Read the model definition and answer for the solid it produces. Units are mm, in the model's axes. A direction names the side the tool comes from. Coordinates: 2 decimals unless noted, no trailing zeros. Order: outer loops, then holes, each group sorted by start corner. A loop starts at its lowest first (then second) coordinate and runs counter-clockwise, first axis right, second up. Notation, with made-up numbers: (46, 50) -> (98, 50) arc R29 cw to (98, 74) -> close; hole circle Ø10 at (-35.5, -19.5). An arc over 180 degrees is marked (long way). Answer in a Markdown table with one row per item.
from build123d import *

# Parameters (mm, degrees)
FACE_SKETCH_W                       = 145.5
FACE_SKETCH_H                       = 95.5
FACE_SKETCH_R                       = 0.5
FACE_SKETCH_R_2                     = 2.5
FACE_SKETCH_R_3                     = 4
FACE_SKETCH_W_2                     = 80.6
FACE_SKETCH_H_2                     = 53.2
FACE_EXTRUDE_DEPTH                  = 2.25
SKETCH1_R                           = 11.375
STOP_BUTTON_MOUNTING_HOLE_CUT_DEPTH = 107.125809773
WALLS_SKETCH_W                      = 145.5
WALLS_SKETCH_H                      = 95.5
WALLS_SKETCH_W_2                    = 141
WALLS_SKETCH_H_2                    = 91
WALLS_EXTRUDE_DEPTH                 = 21.25
SD_CARD_ACCESS_SKETCH_W             = 9.5
SD_CARD_ACCESS_SKETCH_H             = 31
SD_CARD_CUT_DEPTH                   = 2.5
EDGE_RADIUS_R                       = 2
TOP_CONNECTORS_CUT_DEPTH            = 109.208999164
TOP_CONNECTORS_CUT_DEPTH_BACK       = 109.208999164
TOP_CONNECTORS_SKETCH_R             = 1.6


with BuildPart() as part:
    # Face Sketch → Face Extrude (new body)
    with BuildSketch(Plane.XY):
        with Locations((22, 0)):
            Rectangle(FACE_SKETCH_W, FACE_SKETCH_H)
        with Locations((18.7, -35.5)):
            Circle(FACE_SKETCH_R, mode=Mode.SUBTRACT)
        with Locations((3.5, -35.5)):
            Circle(FACE_SKETCH_R_2, mode=Mode.SUBTRACT)
        with Locations((36.5, -35.5)):
            Circle(FACE_SKETCH_R_3, mode=Mode.SUBTRACT)
        with Locations((18.7, -32)):
            Circle(FACE_SKETCH_R, mode=Mode.SUBTRACT)
        with Locations((21.731088913, -33.75)):
            Circle(FACE_SKETCH_R, mode=Mode.SUBTRACT)
        with Locations((21.731088913, -37.25)):
            Circle(FACE_SKETCH_R, mode=Mode.SUBTRACT)
        with Locations((18.7, -39)):
            Circle(FACE_SKETCH_R, mode=Mode.SUBTRACT)
        with Locations((15.668911087, -37.25)):
            Circle(FACE_SKETCH_R, mode=Mode.SUBTRACT)
        with Locations((15.668911087, -33.75)):
            Circle(FACE_SKETCH_R, mode=Mode.SUBTRACT)
        with Locations((0, 8.6)):
            Rectangle(FACE_SKETCH_W_2, FACE_SKETCH_H_2, mode=Mode.SUBTRACT)
    extrude(amount=FACE_EXTRUDE_DEPTH)

    # Sketch1 → Stop Button Mounting Hole Cut (cut, through all)
    with BuildSketch(Plane.XY):
        with Locations((72.75, 0)):
            Circle(SKETCH1_R)
    extrude(amount=STOP_BUTTON_MOUNTING_HOLE_CUT_DEPTH, mode=Mode.SUBTRACT)

    # Walls Sketch → Walls Extrude (add)
    with BuildSketch(Plane(origin=(0, 0, 0), x_dir=(-1, 0, 0), z_dir=(0, 0, -1))):
        with Locations((-22, 0)):
            Rectangle(WALLS_SKETCH_W, WALLS_SKETCH_H)
        with Locations((-22, 0)):
            Rectangle(WALLS_SKETCH_W_2, WALLS_SKETCH_H_2, mode=Mode.SUBTRACT)
    extrude(amount=WALLS_EXTRUDE_DEPTH)

    # SD Card Access Sketch → SD Card Cut (cut)
    with BuildSketch(Plane.ZY.offset(50.75)):
        with Locations((-16.5, 7.5)):
            Rectangle(SD_CARD_ACCESS_SKETCH_W, SD_CARD_ACCESS_SKETCH_H)
    extrude(amount=-SD_CARD_CUT_DEPTH, mode=Mode.SUBTRACT)

    # Edge Radius
    edge_radius_edges = [part.edges().sort_by_distance(p)[0] for p in [
        (94.75, 0, 2.25),
        (22, 47.75, 2.25),
        (-50.75, 0, 2.25),
        (22, -47.75, 2.25),
        (-50.75, 47.75, -9.5),
        (94.75, 47.75, -9.5),
        (94.75, -47.75, -9.5),
        (-50.75, -47.75, -9.5),
    ]]
    fillet(edge_radius_edges, radius=EDGE_RADIUS_R)

    # Top Connectors Sketch → Top Connectors Cut (cut, two sides: drawn at the far end of the back side and taken through both)
    with BuildSketch(Plane(origin=(0, 0, 0), x_dir=(0, 0, -1), z_dir=(1, 0, 0)).offset(-TOP_CONNECTORS_CUT_DEPTH_BACK)):
        with Locations((15.625, 35)):
            Circle(TOP_CONNECTORS_SKETCH_R)
        with Locations((15.625, -18)):
            Circle(TOP_CONNECTORS_SKETCH_R)
    extrude(amount=TOP_CONNECTORS_CUT_DEPTH + TOP_CONNECTORS_CUT_DEPTH_BACK, mode=Mode.SUBTRACT)


solid = part.part
Q1. The part is cut by section C-C (y = 0). Write down the section's boundary in (x, z) (3 decimals), then the cut area to 3 significant figures.
Outcome:
| item | result |
|---|---|
| outline | (-50.75, -11.75) -> (-48.5, -11.75) -> (-48.5, 0) -> (-40.3, 0) -> (-40.3, 2.25) -> (-48.75, 2.25) arc R2 ccw to (-50.75, 0.25) -> close; (40.3, 0) -> (61.375, 0) -> (61.375, 2.25) -> (40.3, 2.25) -> close; (84.125, 0) -> (92.5, 0) -> (92.5, -21.25) -> (94.75, -21.25) -> (94.75, 0.25) arc R2 ccw to (92.75, 2.25) -> (84.125, 2.25) -> close |
| area | 167 mm² |
Q2. For a pull along X with two mould halves and no side action, classify faces 3 (the face through (23, 45.5, -10)), 4 (the face through (94.75, -1, -10)), 5 (the face through (93.609, -16.919, -14.446)) as pulls with the +X half, pulls with the -X half, needs draft (parallel to the pull), parting line crosses it, or undercut.
Outcome:
| item | result |
|---|---|
| face 3 | undercut |
| face 4 | pulls with the +X half |
| face 5 | needs draft |
Q3. For faces 1 (the face through (22, 46, -21.25)), 2 (the face through (21, -20, 0)), determine the directions among +Z, -Z, +X, -X, +Y, -Y from which every point of the face is accessible in a straight line to the end or side of a thin tool.
Outcome:
| item | result |
|---|---|
| face 1 | -Z, +X, -X, +Y, -Y |
| face 2 | -Z |
Q4. Given pin 1 (12 mm diameter, centred on x = 79.5, y = -22.5, fed in from -Z); pin 2 (0.7 mm diameter, centred on y = 3, z = 1.5, fed in from -X); pin 3 (0.7 mm diameter, centred on x = -50, z = -16.5, fed in from +Y), each flat-ended and moving along its own axis, determine where each tip first touches the part or whether it passes through.
Outcome:
| item | result |
|---|---|
| pin 1 | z = 0 |
| pin 2 | x = -50.54 |
| pin 3 | y = 47.54 |
Q5. Consider line 1 (X direction, y = -21, z = -12); line 2 (Y direction, x = 18.7, z = 1.75); line 3 (Y direction, x = 18.7, z = 1.6). Determine where each line is inside the solid, lowest interval first.
Outcome:
| item | result |
|---|---|
| line 1 | -50.75 to -48.5, 92.5 to 94.75 |
| line 2 | -47.07 to -39.5, -38.5 to -36, -35 to -32.5, -31.5 to -18, 35.2 to 47.07 |
| line 3 | -47.23 to -39.5, -38.5 to -36, -35 to -32.5, -31.5 to -18, 35.2 to 47.23 |
Q6. The part is cut by section B-B (x = 3.5). Write down the section's boundary in (y, z).
Outcome:
| item | result |
|---|---|
| outline | (-47.75, -21.25) -> (-45.5, -21.25) -> (-45.5, 0) -> (-38, 0) -> (-38, 2.25) -> (-45.75, 2.25) arc R2 ccw to (-47.75, 0.25) -> close; (-33, 0) -> (-18, 0) -> (-18, 2.25) -> (-33, 2.25) -> close; (35.2, 0) -> (45.5, 0) -> (45.5, -21.25) -> (47.75, -21.25) -> (47.75, 0.25) arc R2 ccw to (45.75, 2.25) -> (35.2, 2.25) -> close |
Q7. The part is cut by section D-D (z = -3.5). Write down the section's boundary in (x, y).
Outcome:
| item | result |
|---|---|
| outline | (-50.75, -45.75) arc R2 ccw to (-48.75, -47.75) -> (92.75, -47.75) arc R2 ccw to (94.75, -45.75) -> (94.75, 45.75) arc R2 ccw to (92.75, 47.75) -> (-48.75, 47.75) arc R2 ccw to (-50.75, 45.75) -> close; hole (-48.5, -45.5) -> (92.5, -45.5) -> (92.5, 45.5) -> (-48.5, 45.5) -> close |
Q8. The part is cut by section A-A (x = 72.75). Write down the section's boundary in (y, z) (3 decimals).
Outcome:
| item | result |
|---|---|
| outline | (-47.75, -21.25) -> (-45.5, -21.25) -> (-45.5, 0) -> (-11.375, 0) -> (-11.375, 2.25) -> (-45.75, 2.25) arc R2 ccw to (-47.75, 0.25) -> close; (11.375, 0) -> (45.5, 0) -> (45.5, -21.25) -> (47.75, -21.25) -> (47.75, 0.25) arc R2 ccw to (45.75, 2.25) -> (11.375, 2.25) -> close |
